from build123d import *

# Parameters (mm, degrees)
F0_R     = 2
F1_DEPTH = 25
F3_DEPTH = 276
F4_R     = 2
F5_DEPTH = 84.8
F6_R     = 2.5
F7_DEPTH = 5


with BuildPart() as f1:
    # F0 (on Top) → F1 (new body)
    with BuildSketch(Plane.XY):
        with BuildLine():
            Line((-51.434658, 66.572686), (-81.434658, 66.572686))
            Line((-81.434658, 66.572686), (-81.434658, -43.427314))
            Line((-81.434658, -43.427314), (-6.434658, -43.427314))
            ThreePointArc((-6.434658, -43.427314), (8.565342, -58.427314), (23.565342, -43.427314))
            Line((23.565342, -43.427314), (98.565342, -43.427314))
            Line((98.565342, -43.427314), (98.565342, 66.572686))
            Line((98.565342, 66.572686), (68.565342, 66.572686))
            ThreePointArc((68.565342, 66.572686), (53.565342, 81.572686), (38.565342, 66.572686))
            Line((38.565342, 66.572686), (-21.434658, 66.572686))
            ThreePointArc((-21.434658, 66.572686), (-36.434658, 81.572686), (-51.434658, 66.572686))
        make_face()
        with Locations((8.565342, -50.927314)):
            Circle(F0_R, mode=Mode.SUBTRACT)
        with Locations((-36.434658, 74.072686)):
            Circle(F0_R, mode=Mode.SUBTRACT)
        with Locations((53.565342, 74.072686)):
            Circle(F0_R, mode=Mode.SUBTRACT)
    extrude(amount=F1_DEPTH)

    # F2 (on face) → F3 (cut)
    with BuildSketch(Plane.YZ.offset(98.565342)):
        with BuildLine():
            Line((43.145373, 0), (22.822686, 0))
            ThreePointArc((22.822686, 0), (11.572686, 11.25), (0.322686, 0))
            Line((0.322686, 0), (-20, 0))
            ThreePointArc((-20, 0), (-41.231841, 11.150842), (-64.902842, 15))
            Line((-64.902842, 15), (-64.902842, -16.413443))
            Line((-64.902842, -16.413443), (88.048215, -16.413443))
            Line((88.048215, -16.413443), (88.048215, 15))
            ThreePointArc((88.048215, 15), (64.377213, 11.150842), (43.145373, 0))
        make_face()
    extrude(amount=-F3_DEPTH, mode=Mode.SUBTRACT)

    # F4 (on face) → F5 (cut)
    with BuildSketch(Plane.XY.offset(25)):
        with Locations((-56.434658, 32.872686)):
            Circle(F4_R)
        with Locations((73.565342, 32.872686)):
            Circle(F4_R)
        with Locations((-56.434658, -9.727314)):
            Circle(F4_R)
        with Locations((73.565342, -9.727314)):
            Circle(F4_R)
    extrude(amount=-F5_DEPTH, mode=Mode.SUBTRACT)

    # F6 (on face) → F7 (cut)
    with BuildSketch(Plane.XY.offset(25)):
        with Locations((-56.434658, 32.872686)):
            Circle(F6_R)
        with Locations((73.565342, 32.872686)):
            Circle(F6_R)
        with Locations((73.565342, -9.727314)):
            Circle(F6_R)
        with Locations((-56.434658, -9.727314)):
            Circle(F6_R)
    extrude(amount=-F7_DEPTH, mode=Mode.SUBTRACT)


solid = f1.part
Geometry check sheet. Reference: the model listing, model coordinates, mm. A direction names the side the tool comes from. Give positions to 0.01 mm unless a question says otherwise; leave off trailing zeros. Loops run counter-clockwise (first coordinate to the right, second up) from the corner with the lowest first, then second, coordinate; pieces in that order, holes last.
(1) Depth check by flat-ended pin: pin 1 Ø14.5 at (x, z) = (47.5, 16) entering from -Y; pin 2 Ø4 at (x, y) = (-57, -9.5) entering from +Z; pin 3 Ø4.5 at (x, y) = (73.57, -9.73) entering from +Z; pin 4 Ø6.5 at (x, z) = (-71.5, 20) entering from +Y. Enter the tip coordinate at first touch or a pass-through.
From the geometry:
pin 1: stops at y = -43.43
pin 2: stops at z = 25
pin 3: stops at z = 20
pin 4: stops at y = 66.57
(2) Set-up check for faces 4 (the flat face through (61, -43.427, 18)), 5 (the flat face through (-66, 66.573, 18)), 6 (the flat face through (-58, -8, 20)): record each of +Z, -Z, +X, -X, +Y, -Y from which the full face is reachable in a straight line by a thin tool's end or side.
From the geometry:
face 4: +Z, -Z, +X, -Y
face 5: +Z, -Z, -X, +Y
face 6: +Z
(3) Section check B-B on z = 22.75. Record the cut outline in (x, y).
From the geometry:
outline: (-81.43, -43.43) - (-6.43, -43.43) arc R15 ccw to (23.57, -43.43) - (98.57, -43.43) - (98.57, 66.57) - (68.57, 66.57) arc R15 ccw to (38.57, 66.57) - (-21.43, 66.57) arc R15 ccw to (-51.43, 66.57) - (-81.43, 66.57) - close; hole circle Ø5 at (-56.43, -9.73); hole circle Ø5 at (-56.43, 32.87); hole circle Ø4 at (-36.43, 74.07); hole circle Ø4 at (8.57, -50.93); hole circle Ø4 at (53.57, 74.07); hole circle Ø5 at (73.57, -9.73); hole circle Ø5 at (73.57, 32.87)
(4) Section check A-A on x = 33.5. Record the cut outline in (y, z), then the cut area to 3 significant figures.
From the geometry:
outline: (-43.43, 11.85) arc R74.71 cw to (-20, 0) - (0.32, 0) arc R11.25 cw to (22.82, 0) - (43.15, 0) arc R74.71 cw to (66.57, 11.85) - (66.57, 25) - (-43.43, 25) - close
area: 2,230 mm2
(5) Section check C-C on y = 6.5. Record the cut outline in (x, z), then the cut area to 3 significant figures.
From the geometry:
outline: (-81.43, 10.04) - (98.57, 10.04) - (98.57, 25) - (-81.43, 25) - close
area: 2,690 mm2
(6) Release check for a two-part mould opening along X. For faces 1 (the flat face through (-81.435, 12, 15)), 2 (the cylindrical face through (9.83, 57.32, 8.39)), 3 (the cylindrical face through (53.13, 72.12, 19.05)) record: released by +X, released by -X, zero draft, split by the parting line, or undercut.
From the geometry:
face 1: released by -X
face 2: zero draft
face 3: undercut
(7) Section check D-D on y = -22. Record the cut outline in (x, z).
From the geometry:
outline: (-81.43, 1.45) - (98.57, 1.45) - (98.57, 25) - (-81.43, 25) - close
(8) Thickness scan on L1, parallel to Y at x = 27.5, z = 1.5; L2, parallel to X at y = -44, z = 22.5; L3, parallel to Y at x = -55.5, z = 22.75. Record the ranges inside material, lowest first.
From the geometry:
L1: y = -22.07 to 0.42, 22.72 to 45.21
L2: x = -6.42 to 23.55
L3: y = -43.43 to -12.05, -7.41 to 30.55, 35.19 to 66.57
